For this review, take the finished solid that the model builds, in its own axes (mm). Face numbers are marked on the shaded views. A direction names the side the tool comes from. Coordinates: 2 decimals unless noted, no trailing zeros. Loops run counter-clockwise (first coordinate to the right, second up) from the corner with the lowest first, then second, coordinate; pieces in that order, holes last. Notation, with made-up numbers: (-31, 51.5) -> (-25, 51.5) arc R25 cw to (-25, 68.5) -> close; hole circle Ø4 at (58, 80). An arc over 180 degrees is marked (long way). One line per item, written item: value.
Autodesk Inventor part; units mm, degrees
ref_plane "YZ Plane" through (0, 0, 0) normal (1, 0, 0) x (0, 1, 0)
ref_plane "XZ Plane" through (0, 0, 0) normal (0, 1, 0) x (-1, 0, 0)
ref_plane "XY Plane" through (0, 0, 0) normal (0, 0, 1) x (1, 0, 0)
sketch "Sketch1" plane through (0, 0, 0) normal (0, 0, 1) x (1, 0, 0)
  line L0 (44.453, 0) -> (22.2265, -38.4974)
  line L1 (22.2265, -38.4974) -> (-22.2265, -38.4974)
  line L2 (-22.2265, -38.4974) -> (-44.453, 0)
  line L3 (-44.453, 0) -> (-22.2265, 38.4974)
  line L4 (-22.2265, 38.4974) -> (22.2265, 38.4974)
  line L5 (22.2265, 38.4974) -> (44.453, 0)
  line L6 (22.2265, 38.4974) -> (123, 38.4974)
  line L7 (22.2265, -38.4974) -> (123, -38.4974)
  line L8 (123, -38.4974) -> (123, 38.4974)
  point P0 (0, 0)
  point P1 (0, 0)
  dimension "d1" = 145.2265
  dimension "d2" = 76.9948
extrude "Extrusion1" add sketch "Sketch1" along normal blind 15
sketch "Sketch2" plane through (123, -38.4974, 0) normal (1, 0, 0) x (0, 0, -1)
  circle A0 centre (-7.5, 65.9974) radius 2.5
  circle A1 centre (-7.5, 10.9974) radius 2.5
  line L0 (-7.5, 65.9974) -> (-7.5, 10.9974) construction
  line L1 (0, 0) -> (0, 76.9948) construction
  line L2 (0, 76.9948) -> (-15, 76.9948) construction
  point P0 (0, 38.4974)
  point P1 (-7.5, 38.4974)
  point P2 (0, 38.4974)
  point P3 (-7.5, 76.9948)
  dimension "d5" = 5
  dimension "d6" = 5
  dimension "d7" = 55
extrude "Extrusion2" cut sketch "Sketch2" against normal blind 25
sketch "Sketch3" plane through (0, 0, 0) normal (0, 0, -1) x (-1, 0, 0)
  line L0 (-123, -38.4974) -> (-123, 38.4974)
  line L1 (-123, 7.5) -> (-108, 7.5)
  line L2 (-108, 7.5) -> (-108, -7.5)
  line L3 (-108, -7.5) -> (-123, -7.5)
  line L4 (-123, -7.5) -> (-123, 7.5)
  line L5 (-123, 38.4974) -> (22.2265, 38.4974)
  line L6 (22.2265, 38.4974) -> (44.453, 0)
  line L7 (44.453, 0) -> (22.2265, -38.4974)
  line L8 (22.2265, -38.4974) -> (-123, -38.4974)
  line L9 (38.6795, 0) -> (19.3397, 33.4974)
  line L10 (19.3397, 33.4974) -> (-118, 33.4974)
  line L11 (-118, 33.4974) -> (-118, -33.4974) construction
  line L12 (-118, -33.4974) -> (19.3397, -33.4974)
  line L13 (19.3397, -33.4974) -> (38.6795, 0)
  line L14 (-108, 7.5) -> (-108, 33.4974)
  line L15 (-108, -7.5) -> (-108, -33.4974)
  line L16 (19.3397, 33.4974) -> (-108, 33.4974)
  line L17 (-108, -33.4974) -> (19.3397, -33.4974)
  point P0 (0, 0)
  point P1 (-123, 0)
  dimension "d10" = 15
  dimension "d11" = 15
  dimension "d12" = 5
extrude "Extrusion3" cut sketch "Sketch3" against normal blind 10 contours L0 L1 L2 L3 | L2 L14 L10 L9 L13 L12 L15
sketch "Sketch5" plane through (0, 0, 15) normal (0, 0, 1) x (1, 0, 0)
  line L0 (123, 38.4974) -> (-22.2265, 38.4974)
  line L1 (-22.2265, 38.4974) -> (-44.453, 0)
  line L2 (-44.453, 0) -> (-22.2265, -38.4974)
  line L3 (-22.2265, -38.4974) -> (123, -38.4974)
  line L4 (123, -38.4974) -> (123, 38.4974)
  line L5 (122.5, -37.9974) -> (-21.9378, -37.9974)
  line L6 (-21.9378, -37.9974) -> (-43.8756, 0)
  line L7 (-43.8756, 0) -> (-21.9378, 37.9974)
  line L8 (-21.9378, 37.9974) -> (122.5, 37.9974)
  line L9 (122.5, 37.9974) -> (122.5, -37.9974)
  point P0 (0, 0)
  dimension "d15" = 0.5
extrude "Extrusion4" cut sketch "Sketch5" against normal through all
sketch "Sketch6" plane through (0, 0, 15) normal (0, 0, 1) x (1, 0, 0)
  line L0 (122.5, -37.9974) -> (122.5, 37.9974)
  line L1 (122.5, 37.9974) -> (-21.9378, 37.9974)
  line L2 (-21.9378, 37.9974) -> (-43.8756, 0)
  line L3 (-43.8756, 0) -> (-21.9378, -37.9974)
  line L4 (-21.9378, -37.9974) -> (122.5, -37.9974)
  point P0 (0, 0)
extrude "Extrusion5" add sketch "Sketch6" along normal blind 10
sketch "Sketch7" plane through (0, 0, 10) normal (0, 0, -1) x (-1, 0, 0)
  line L0 (-122.5, 7.5) -> (-122.5, -7.5)
  line L1 (-108, -7.5) -> (-122.5, -7.5)
  line L2 (-108, -27.5) -> (-108, -7.5)
  line L3 (-108, -33.4974) -> (-108, -27.5)
  line L4 (19.3397, -33.4974) -> (-108, -33.4974)
  line L5 (38.6795, 0) -> (19.3397, -33.4974)
  line L6 (19.3397, 33.4974) -> (38.6795, 0)
  line L7 (-108, 33.4974) -> (19.3397, 33.4974)
  line L8 (-108, 27.5) -> (-108, 33.4974)
  line L9 (-108, 7.5) -> (-108, 27.5)
  line L10 (-122.5, 7.5) -> (-108, 7.5)
  line L11 (-108, 7.5) -> (-108, 27.5)
  line L12 (-108, -27.5) -> (-108, -7.5)
  line L13 (-108, 7.5) -> (-108, -7.5)
  point P0 (0, 0)
extrude "Extrusion6" cut sketch "Sketch7" against normal blind 10 contours L9 L8 L7 L6 L5 L4 L3 L2 L13
properties part number "TARM06" material "ABS Plastic"
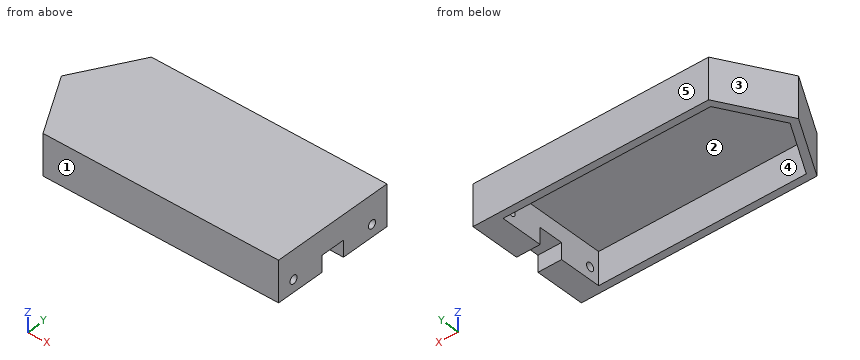
1. Insertion check: pin 1 Ø4 at (y, z) = (27.5, 7.5) entering from +X; pin 2 Ø8 at (x, y) = (68, 26.5) entering from -Z; pin 3 Ø4 at (y, z) = (17, 10.5) entering from -X. Each pin has a flat end and moves straight along its axis. Give the tip position at first contact, or say it passes through.
Return value:
pin 1: stops at x = -21.65
pin 2: stops at z = 20
pin 3: stops at x = -35.22
2. For the marked faces 4 and 5, list the 3-axis set-ups (+Z, -Z, +X, -X, +Y, -Y) from which the entire face can be reached by the end or side of a thin tool; tool diameter is ignored.
Return value:
face 4: -Z
face 5: +Z, -Z, +X, -X, +Y
3. The part is to be moulded in two halves that separate along X. For the marked faces 1, 2 and 3, say which applies: pulls with the +X half, pulls with the -X half, needs draft (parallel to the pull), parting line crosses it, or undercut.
Return value:
face 1: needs draft
face 2: undercut
face 3: pulls with the -X half
4. Take a section at D-D, the plane y = 1.5. Give the boundary of the cut face in (x, z).
Return value:
outline: (-43.01, 0) -> (-37.81, 0) -> (-37.81, 20) -> (108, 20) -> (108, 10) -> (122.5, 10) -> (122.5, 25) -> (-43.01, 25) -> close
5. Take a section at A-A, the plane z = 7.5. Give the boundary of the cut face in (x, y).
Return value:
outline: (-43.88, 0) -> (-21.94, -38) -> (122.5, -38) -> (122.5, -30) -> (108, -30) -> (108, -33.5) -> (-19.34, -33.5) -> (-38.68, 0) -> (-19.34, 33.5) -> (108, 33.5) -> (108, 30) -> (122.5, 30) -> (122.5, 38) -> (-21.94, 38) -> close; (108, -25) -> (122.5, -25) -> (122.5, -7.5) -> (108, -7.5) -> close; (108, 7.5) -> (122.5, 7.5) -> (122.5, 25) -> (108, 25) -> close
6. Take a section at C-C, the plane x = 79. Give the boundary of the cut face in (y, z).
Return value:
outline: (-38, 0) -> (-33.5, 0) -> (-33.5, 20) -> (33.5, 20) -> (33.5, 0) -> (38, 0) -> (38, 25) -> (-38, 25) -> close
7. To check wall thickness, follow probe 1 along Y at (x, z) = (111.75, 7.5); probe 2 along Z at (x, y) = (113.5, -27.5); probe 3 along Y at (x, z) = (91, 6.5). State the ranges of each line that lie inside material, in increasing order. Write a range as from..to.
Return value:
probe 1: y = -38..-30, -25..-7.5, 7.5..25, 30..38
probe 2: z = 0..5, 10..25
probe 3: y = -38..-33.5, 33.5..38
8. Take a section at B-B, the plane y = -27.5. Give the boundary of the cut face in (x, z), and give its area (3 significant figures).
Return value:
outline: (-28, 0) -> (-22.8, 0) -> (-22.8, 20) -> (108, 20) -> (108, 10) -> (122.5, 10) -> (122.5, 25) -> (-28, 25) -> close; (108, 0) -> (122.5, 0) -> (122.5, 5) -> (108, 5) -> close
area: 1,070 mm2
